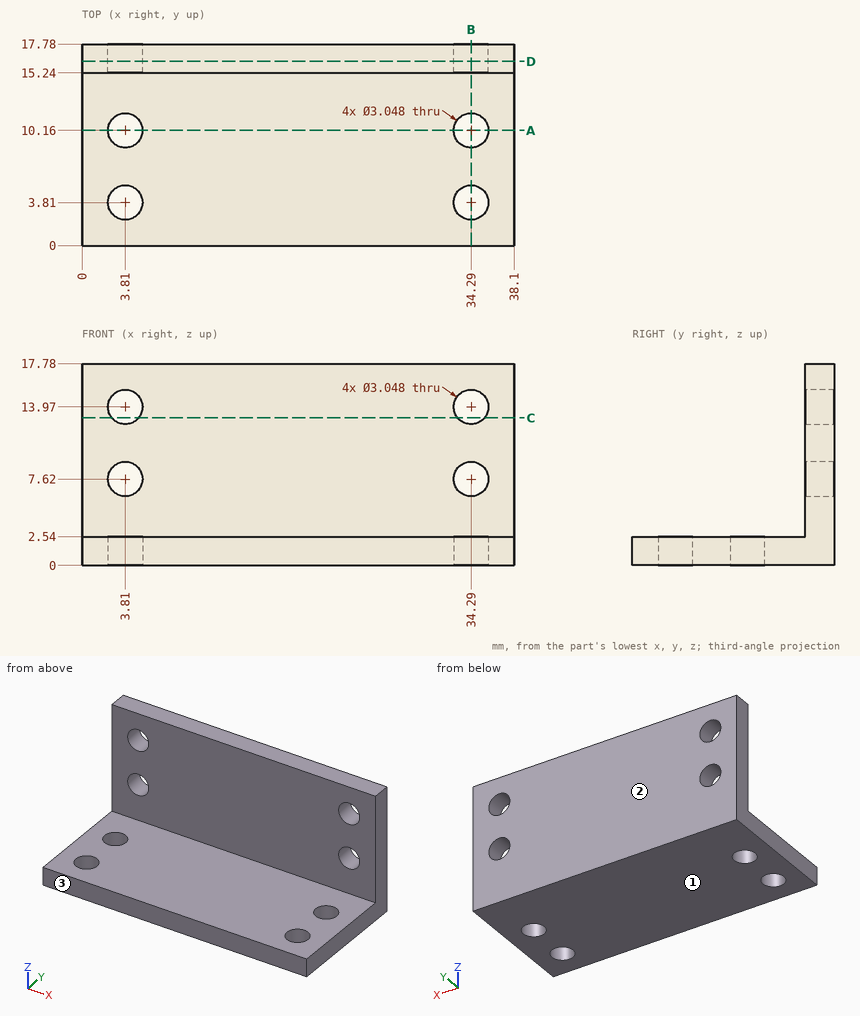
Answer from the drawing. Dimensions are ordinates in mm from the lowest x, y and z of the part. Coordinates: 2 decimals unless noted, no trailing zeros. Loops run counter-clockwise (first coordinate to the right, second up) from the corner with the lowest first, then second, coordinate; pieces in that order, holes last.
Q1. The part is cut by section A-A on y = 10.16. Write down the section's boundary in (x, z).
Q2. The part is cut by section D-D on y = 16.25. Write down the section's boundary in (x, z).
Q3. The part is cut by section B-B on x = 34.29. Write down the section's boundary in (y, z).
Q4. The mould has two halves that part along Y. Classify the marked faces 1, 2 and 3: +Y half, -Y half, draft (parallel to the pull), parting line (faces both ways), or undercut.
Q5. The part is cut by section C-C on z = 13. Write down the section's boundary in (x, y).
Q6. Consider probe 1 along X at (y, z) = (16.25, 13.97); probe 2 along Z at (x, y) = (34.29, 17); probe 3 along Y at (x, z) = (15, 3.75). Determine where each line is inside the solid, lowest interval first.
Q7. Each of these flat-tipped pins is pushed along its axis until it touches: pin 1 Ø8 at (x, y) = (30, 3.5) entering from +Z; pin 2 Ø2.5 at (x, z) = (34.29, 13.97) entering from -Y; pin 3 Ø4.5 at (x, z) = (12.5, 11.5) entering from -Y. Where does it stop, or does it pass through?
Results below:
1. outline: (0, 0) - (2.29, 0) - (2.29, 2.54) - (0, 2.54) - close; (5.33, 0) - (32.77, 0) - (32.77, 2.54) - (5.33, 2.54) - close; (35.81, 0) - (38.1, 0) - (38.1, 2.54) - (35.81, 2.54) - close
2. outline: (0, 0) - (38.1, 0) - (38.1, 17.78) - (0, 17.78) - close; hole circle Ø3.05 at (3.81, 7.62); hole circle Ø3.05 at (3.81, 13.97); hole circle Ø3.05 at (34.29, 7.62); hole circle Ø3.05 at (34.29, 13.97)
3. outline: (0, 0) - (2.29, 0) - (2.29, 2.54) - (0, 2.54) - close; (5.33, 0) - (8.64, 0) - (8.64, 2.54) - (5.33, 2.54) - close; (11.68, 0) - (17.78, 0) - (17.78, 6.1) - (15.24, 6.1) - (15.24, 2.54) - (11.68, 2.54) - close; (15.24, 9.14) - (17.78, 9.14) - (17.78, 12.45) - (15.24, 12.45) - close; (15.24, 15.49) - (17.78, 15.49) - (17.78, 17.78) - (15.24, 17.78) - close
4. face 1: draft
4. face 2: +Y half
4. face 3: -Y half
5. outline: (0, 15.24) - (2.63, 15.24) - (2.63, 17.78) - (0, 17.78) - close; (4.99, 15.24) - (33.11, 15.24) - (33.11, 17.78) - (4.99, 17.78) - close; (35.47, 15.24) - (38.1, 15.24) - (38.1, 17.78) - (35.47, 17.78) - close
6. probe 1: x = 0 to 2.29, 5.33 to 32.77, 35.81 to 38.1
6. probe 2: z = 0 to 6.1, 9.14 to 12.45, 15.49 to 17.78
6. probe 3: y = 15.24 to 17.78
7. pin 1: stops at z = 2.54
7. pin 2: passes through
7. pin 3: stops at y = 15.24
